Here's how the part is built. I have some questions about the finished solid (model axes, mm). Face numbers are marked on the shaded views. A direction names the side the tool comes from. Coordinates: 2 decimals unless noted, no trailing zeros. Write each loop counter-clockwise with the first axis right and the second up, starting at its lowest first coordinate (ties: lowest second). Pieces come first, ordered by that corner, then holes. Notation, with made-up numbers: (6.5, 70) -> (57.5, 70) arc R26 cw to (57.5, 102) -> close; hole circle Ø8 at (-5, 69.25). An arc over 180 degrees is marked (long way). Put each result on its own line as item: value. Start each with the question number.
Item 1: I need wall thicknesses on line 1 (Z direction, x = -20, y = -12.75); line 2 (Y direction, x = -3, z = 17.25); line 3 (X direction, y = -2.25, z = 14.5). Which ranges of each line are inside material? Lowest first, please. Write a range as [from, to].
Item 2: I want a section at B-B, the plane z = 10. List the corners of the cut face in (x, y) for me, then the cut area to 3 significant figures.
Item 3: On a 3-axis mill with a long thin cutter (end or side, diameter ignored), from which of +Z, -Z, +X, -X, +Y, -Y can I reach the whole of each face in a straight line? I mean the marked faces 4 and 5. Say none if no direction works.
Item 4: I want a section at D-D, the plane x = -11.5. List the corners of the cut face in (y, z) for me, then the cut area to 3 significant figures.
Item 5: I want a section at A-A, the plane x = -20. List the corners of the cut face in (y, z) for me, then the cut area to 3 significant figures.
Item 6: For pin 1 (5 mm diameter, centred on y = -3, z = 9.5, fed in from -X); pin 2 (3.5 mm diameter, centred on y = -4, z = 10, fed in from +X), each with a flat end and sliding along its axis, tell me the tip position at first contact or that it passes through.
Item 7: If we mould it in two halves opening along Z, with no side actions, what happens to the marked faces 1, 2 and 3? For each: released by +Z, released by -Z, zero draft, split by the parting line, or undercut.
Item 8: I want a section at C-C, the plane y = -4. List the corners of the cut face in (x, z) for me.
Autodesk Inventor part; units mm, degrees
ref_plane "YZ Plane" through (0, 0, 0) normal (1, 0, 0) x (0, 1, 0)
ref_plane "XZ Plane" through (0, 0, 0) normal (0, 1, 0) x (-1, 0, 0)
ref_plane "XY Plane" through (0, 0, 0) normal (0, 0, 1) x (1, 0, 0)
sketch "Sketch1" plane through (0, 0, 0) normal (0, 0, 1) x (1, 0, 0)
  line L0 (0, 0) -> (-30, 0)
  line L1 (-30, 0) -> (-30, 10)
  line L2 (-30, 10) -> (0, 10)
  line L3 (0, 10) -> (0, 0)
  line L4 (0, 10) -> (12, 10)
  line L5 (12, 10) -> (12, -18)
  line L6 (12, -18) -> (0, -18)
  line L7 (0, -18) -> (0, 10)
  line L8 (0, -18) -> (-30, -18)
  line L9 (-30, -18) -> (-30, -8)
  line L10 (-30, -8) -> (0, -8)
  line L11 (0, -8) -> (0, -18)
  dimension "d0" = 8
  dimension "d1" = 10
  dimension "d2" = 10
  dimension "d3" = 12
  dimension "d4" = 30
extrude "Extrusion1" add sketch "Sketch1" along normal blind 20
sketch "Sketch2" plane through (0, -8, 0) normal (-1, 0, 0) x (0, 0, 1)
  line L0 (20, 8) -> (20, 0)
  line L1 (0, 8) -> (0, 0)
  line L2 (0, 4) -> (20, 4) construction
  circle A0 centre (10, 4) radius 3.05
  dimension "d7" = 6.1
extrude "Extrusion2" cut sketch "Sketch2" against normal through all
sketch "Sketch3" plane through (-30, 10, 0) normal (0, 1, 0) x (1, 0, 0)
  line L0 (30, 0) -> (30, -20)
  line L1 (30, -10) -> (10, -10) construction
  circle A0 centre (10, -10) radius 3.05
  circle A1 centre (10, -10) radius 8.5 construction
  line L2 (42, 0) -> (42, -20)
  dimension "d10" = 17
  dimension "d11" = 6.1
  dimension "d12" = 20
  dimension "d24" = 11.5
  dimension "d25" = 32
extrude "Extrusion3" cut sketch "Sketch3" against normal through all
sketch "Sketch4" plane through (-30, 0, 0) normal (-1, 0, 0) x (0, 0, 1)
  circle A0 centre (10, -4) radius 3.05
  circle A1 centre (10, -4) radius 5
  dimension "d15" = 10
extrude "Extrusion4" cut sketch "Sketch4" against normal up to surface (30 mm away)
chamfer "Chamfer1" distance 6 angle 45 4 edges at (-30, 5, 0) (-30, 5, 20) (-30, -13, 0) (-30, -13, 20)
chamfer "Chamfer2" distance 6 angle 45 2 edges at (12, 10, 10) (12, -18, 10)
properties part number "cross head"
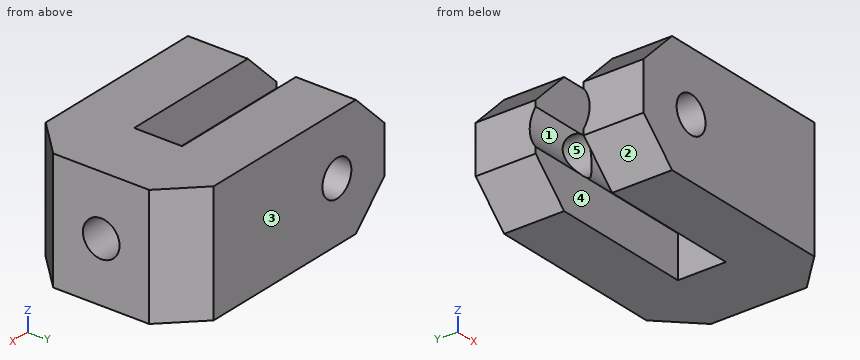
Calculated:
1. line 1: z = [0, 6.95], [13.05, 20]
1. line 2: y = [-18, -8], [0, 10]
1. line 3: x = [0, 12]
2. outline: (-30, -18) -> (-23.05, -18) -> (-23.05, -9) -> (-30, -9) -> close; (-30, 1) -> (-23.05, 1) -> (-23.05, 10) -> (-30, 10) -> close; (-16.95, -18) -> (6, -18) -> (12, -12) -> (12, -7.05) -> (0, -7.05) -> (0, -9) -> (-16.95, -9) -> close; (-16.95, 1) -> (0, 1) -> (0, -0.95) -> (12, -0.95) -> (12, 4) -> (6, 10) -> (-16.95, 10) -> close
2. area: 657 mm2
3. face 4: +Z, -Z, -X
3. face 5: +Y, -Y
4. outline: (-18, 0) -> (-8, 0) -> (-8, 7) arc R5 cw to (-8, 13) -> (-8, 20) -> (-18, 20) -> close; (0, 0) -> (10, 0) -> (10, 20) -> (0, 20) -> (0, 13) arc R5 cw to (0, 7) -> close
4. area: 392 mm2
5. outline: (-18, 0) -> (-8, 0) -> (-8, 6.95) -> (-18, 6.95) -> close; (-18, 13.05) -> (-8, 13.05) -> (-8, 20) -> (-18, 20) -> close; (0, 0) -> (10, 0) -> (10, 6.95) -> (0, 6.95) -> close; (0, 13.05) -> (10, 13.05) -> (10, 20) -> (0, 20) -> close
5. area: 278 mm2
6. pin 1: stops at x = 0
6. pin 2: passes through
7. face 1: undercut
7. face 2: released by -Z
7. face 3: zero draft
8. outline: (0, 0) -> (12, 0) -> (12, 6.95) -> (0, 6.95) -> close; (0, 13.05) -> (12, 13.05) -> (12, 20) -> (0, 20) -> close
